Study the drawing (mm; zero at the part's minimum x, y, z) and answer. Coordinates: 2 decimals unless noted, no trailing zeros. Order: outer loops, then holes, each group sorted by start corner. A loop starts at its lowest first (then second) coordinate and runs counter-clockwise, first axis right, second up.
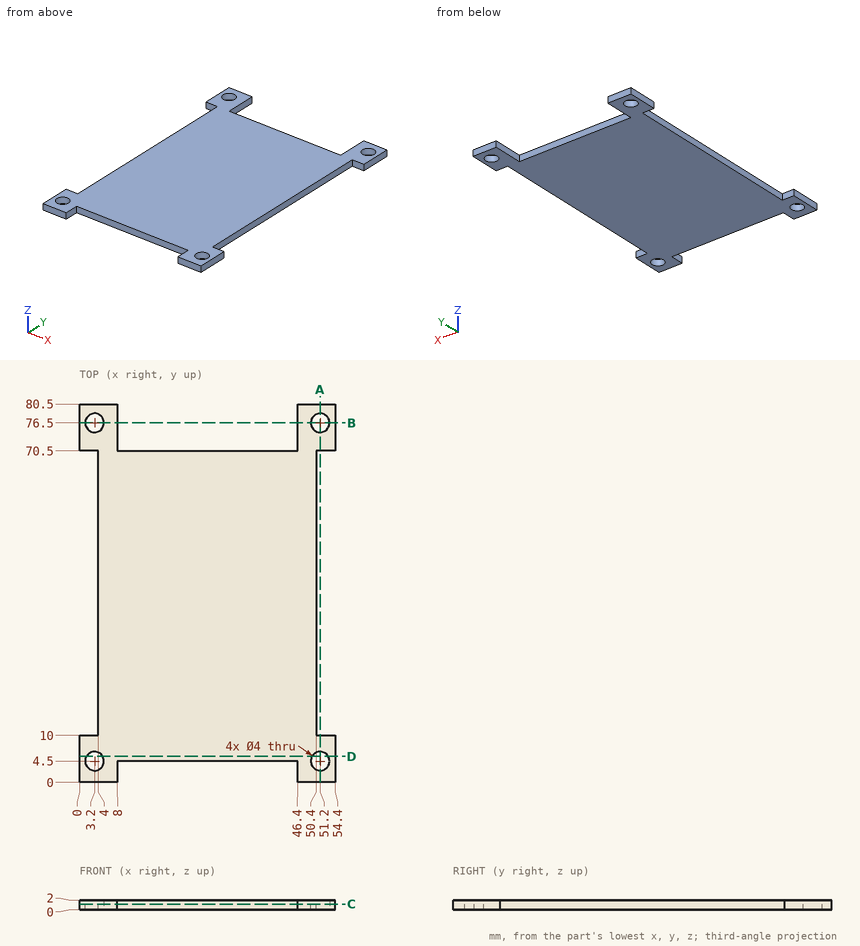
(1) Find section C-C on z = 1.2. Determine the outline of the cut face in (x, y), then the cut area to 3 significant figures.
(2) Find section A-A on x = 51.2. Determine the outline of the cut face in (y, z), then the cut area to 3 significant figures.
(3) Given pin 1 Ø0.6 at (x, z) = (36, 1) entering from +Y; pin 2 Ø0.6 at (x, z) = (28, 1) entering from -Y, each flat-ended and moving along its own axis, determine where each tip first touches the part or whether it passes through.
(4) Find section B-B on y = 76.5. Determine the outline of the cut face in (x, z).
(5) Find section D-D on y = 5.5. Determine the outline of the cut face in (x, z), then the cut area to 3 significant figures.
(6) Find the intervals of material crossed by probe 1 along Y at (x, z) = (3.2, 0.9); probe 2 along Y at (x, z) = (5, 1.6); probe 3 along X at (y, z) = (71.5, 0.55), in increasing order.
Resolved:
1. outline: (0, 0) - (8, 0) - (8, 4.5) - (46.4, 4.5) - (46.4, 0) - (54.4, 0) - (54.4, 10) - (50.4, 10) - (50.4, 70.5) - (54.4, 70.5) - (54.4, 80.5) - (46.4, 80.5) - (46.4, 70.5) - (8, 70.5) - (8, 80.5) - (0, 80.5) - (0, 70.5) - (4, 70.5) - (4, 10) - (0, 10) - close; hole circle Ø4 at (3.2, 4.5); hole circle Ø4 at (3.2, 76.5); hole circle Ø4 at (51.2, 4.5); hole circle Ø4 at (51.2, 76.5)
1. area: 3,290 mm2
2. outline: (0, 0) - (2.5, 0) - (2.5, 2) - (0, 2) - close; (6.5, 0) - (10, 0) - (10, 2) - (6.5, 2) - close; (70.5, 0) - (74.5, 0) - (74.5, 2) - (70.5, 2) - close; (78.5, 0) - (80.5, 0) - (80.5, 2) - (78.5, 2) - close
2. area: 24.0 mm2
3. pin 1: stops at y = 70.5
3. pin 2: stops at y = 4.5
4. outline: (0, 0) - (1.2, 0) - (1.2, 2) - (0, 2) - close; (5.2, 0) - (8, 0) - (8, 2) - (5.2, 2) - close; (46.4, 0) - (49.2, 0) - (49.2, 2) - (46.4, 2) - close; (53.2, 0) - (54.4, 0) - (54.4, 2) - (53.2, 2) - close
5. outline: (0, 0) - (1.47, 0) - (1.47, 2) - (0, 2) - close; (4.93, 0) - (49.47, 0) - (49.47, 2) - (4.93, 2) - close; (52.93, 0) - (54.4, 0) - (54.4, 2) - (52.93, 2) - close
5. area: 94.9 mm2
6. probe 1: y = 0 to 2.5, 6.5 to 10, 70.5 to 74.5, 78.5 to 80.5
6. probe 2: y = 0 to 3.63, 5.37 to 75.63, 77.37 to 80.5
6. probe 3: x = 0 to 8, 46.4 to 54.4
